Study the drawing (mm; zero at the part's minimum x, y, z) and answer. Round coordinates to 2 decimals unless told otherwise and drop trailing zeros. Write each loop counter-clockwise with the first axis right and the second up, starting at its lowest first coordinate (ties: lowest second). Pieces come first, ordered by that corner, then holes.
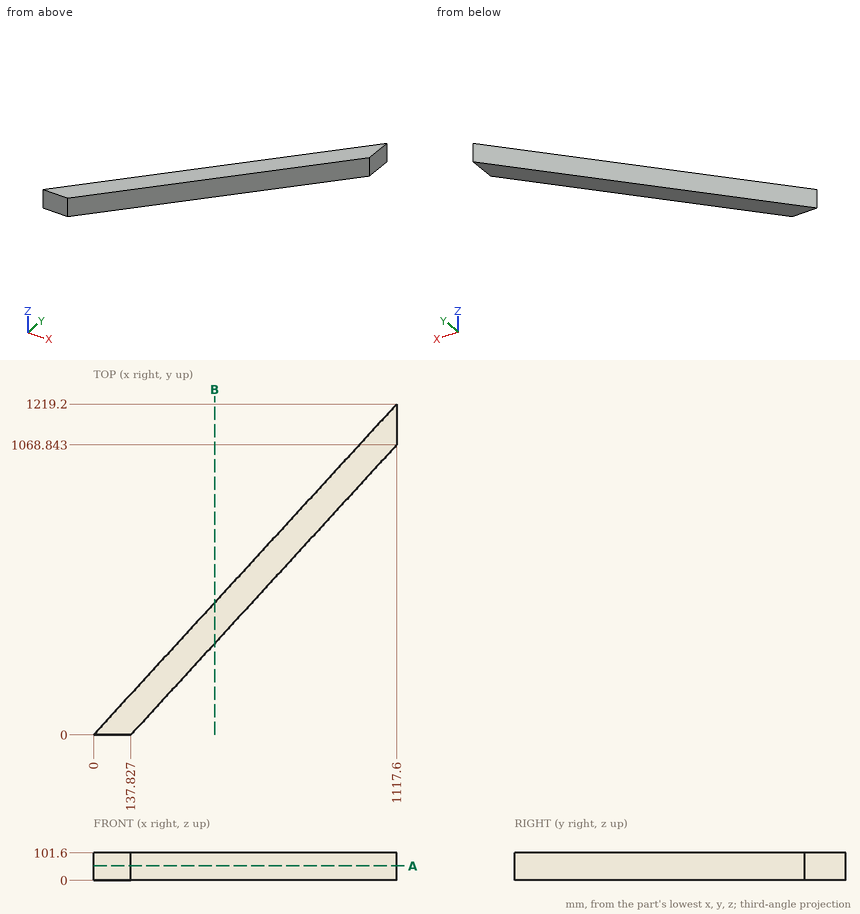
Q1. Given pin 1 (3 mm diameter, centred on x = 478.5, z = 29.5, fed in from -Y) (1 decimal); pin 2 (3 mm diameter, centred on y = 684, z = 43, fed in from +X); pin 3 (3 mm diameter, centred on x = 662.5, z = 23.5, fed in from +Y) (1 decimal), each flat-ended and moving along its own axis, determine where each tip first touches the part or whether it passes through.
Q2. Find the intervals of material crossed by L1, parallel to Y at x = 622, z = 89 (1 decimal); L2, parallel to Y at x = 709.5, z = 25 (1 decimal); L3, parallel to X at y = 302.5, z = 48, in increasing order.
Q3. Find section A-A (z = 53). Determine the outline of the cut face in (x, y), plus the area to 3 significant figures.
Q4. Find section B-B (x = 446.5). Determine the outline of the cut face in (y, z), plus the area to 3 significant figures.
Report:
1. pin 1: stops at y = 370
1. pin 2: stops at x = 766.2
1. pin 3: stops at y = 724.4
2. L1: y = 528.2 to 678.5
2. L2: y = 623.6 to 774
2. L3: x = 277.29 to 415.12
3. outline: (0, 0) - (137.83, 0) - (1117.6, 1068.84) - (1117.6, 1219.2) - close
3. area: 158,000 mm2
4. outline: (336.73, 0) - (487.09, 0) - (487.09, 101.6) - (336.73, 101.6) - close
4. area: 15,300 mm2
